Work out the finished part from the listing and answer in its coordinate system (mm). A direction names the side the tool comes from. Coordinates: 2 decimals unless noted, no trailing zeros. Order: outer loops, then holes, each group sorted by start corner. A loop starts at its lowest first (then second) coordinate and runs counter-clockwise, first axis right, second up.
1. The part is cut by section A-A, the plane z = -191. Give the vertices of the cut face in (x, y), then the cut area to 3 significant figures.
2. Flat-ended cylindrical pins translate along their axes: pin 1 Ø12 at (x, z) = (14, 3.5) entering from -Y; pin 2 Ø3 at (y, z) = (-79.5, -268.5) entering from -X; pin 3 Ø1.5 at (y, z) = (80, -9) entering from -X. Find the tip coordinate at first contact, or state that the pin passes through.
3. A tool of negligible diameter and unlimited length cuts with its end or side. For faces 1 (the flat face through (-345, -50, -250.774)), 2 (the flat face through (-38.1, -51, -160)), 3 (the flat face through (10, 85, 0)), 4 (the flat face through (-660.4, -50, -127)), 5 (the flat face through (-139.7, -18, -33)), from which of +Z, -Z, +X, -X, +Y, -Y can it reach the whole face along a straight path? Write none if from no direction.
4. The part is cut by section D-D, the plane x = -434.5. Give the vertices of the cut face in (y, z).
5. The part is cut by section B-B, the plane y = -45. Give the vertices of the cut face in (x, z).
6. Find the intervals of material crossed by probe 1 along X at (y, z) = (11, -62.5); probe 2 along Z at (x, y) = (-698.5, -65); probe 3 along X at (y, z) = (-39.5, -110), in increasing order.
7. Determine the mould class of faces 6 (the flat face through (10, 0, 84)), 7 (the flat face through (-165.1, -24, -24)), 8 (the flat face through (165.1, -1, -1)), 9 (the flat face through (-408, -76.2, -253)) for opening direction Y: +Y half, -Y half, draft (parallel to the pull), parting line (faces both ways), or undercut.
8. The part is cut by section C-C, the plane y = 55.5. Give the vertices of the cut face in (x, z), then the cut area to 3 significant figures.
```python
from build123d import *

# Parameters (mm, degrees)
F3_R      = 12.7
F4_DEPTH  = 50.8
F4_FACE_W = 76.2
F4_FACE_H = 50.8
F6_W      = 218.9167588949
F6_H      = 225.1323610544
F7_DEPTH  = 723.20793


with BuildPart() as f1:
    # F0 (on Front) → F1 (revolve)
    with BuildSketch(Plane.XZ):
        Polygon((165.1, 76.2), (165.1, 0), (190.5, 0), (190.5, 101.6), (-165.1, 101.6), (-165.1, 25.4), (-139.7, 25.4), (-139.7, 76.2), align=None)
    revolve(axis=Axis((0, 0, 0), (1, 0, 0)))

    # F3 (on offset) → F4 (join)
    with BuildSketch(Plane.XZ.offset(25.4)):
        with BuildLine():
            Line((38.1, -98.3737769937), (-38.1, -98.3737769937))
            Line((-38.1, -98.3737769937), (-38.1, -250.7737769937))
            Line((-38.1, -250.7737769937), (-660.4, -250.7737769937))
            Line((-660.4, -250.7737769937), (-660.4, 0))
            ThreePointArc((-660.4, 0), (-671.5592316368, 26.9407683632), (-698.5, 38.1))
            ThreePointArc((-698.5, 38.1), (-725.4407683632, 26.9407683632), (-736.6, 0))
            Line((-736.6, 0), (-736.6, -326.9737769937))
            Line((-736.6, -326.9737769937), (-660.4, -326.9737769937))
            Line((-660.4, -326.9737769937), (38.1, -326.9737769937))
            Line((38.1, -326.9737769937), (38.1, -250.7737769937))
            Line((38.1, -250.7737769937), (38.1, -98.3737769937))
        make_face()
        with Locations((-698.5, 0)):
            Circle(F3_R, mode=Mode.SUBTRACT)
    extrude(amount=F4_DEPTH)

    # F4_face (on face) → F5 (join, up to the next surface of F1)
    with BuildSketch(Plane(origin=(0, -50.8, -98.3737769937), x_dir=(1, 0, 0), z_dir=(0, 0, 1))):
        Rectangle(F4_FACE_W, F4_FACE_H)
    extrude(until=Until.NEXT)

    # F6 (on face) → F7 (cut)
    with BuildSketch(Plane(origin=(-165.1, 0, 0), x_dir=(0, -1, 0), z_dir=(-1, 0, 0))):
        with Locations((-109.4583794475, 112.5661805272)):
            Rectangle(F6_W, F6_H)
    extrude(amount=-F7_DEPTH, mode=Mode.SUBTRACT)


solid = f1.part
```
Geometry says:
1. outline: (-736.6, -76.2) - (-660.4, -76.2) - (-660.4, -25.4) - (-736.6, -25.4) - close; (-38.1, -76.2) - (38.1, -76.2) - (38.1, -25.4) - (-38.1, -25.4) - close
1. area: 7,740 mm2
2. pin 1: stops at y = -101.6
2. pin 2: passes through
2. pin 3: stops at x = -165.1
3. face 1: +Y, -Y
3. face 2: -Y
3. face 3: +Z, +X, -X, +Y
3. face 4: +Z, +Y, -Y
3. face 5: none
4. outline: (-76.2, -326.97) - (-25.4, -326.97) - (-25.4, -250.77) - (-76.2, -250.77) - close
5. outline: (-736.6, -326.97) - (38.1, -326.97) - (38.1, -91.09) - (190.5, -91.09) - (190.5, 91.09) - (-165.1, 91.09) - (-165.1, -91.09) - (-38.1, -91.09) - (-38.1, -250.77) - (-660.4, -250.77) - (-660.4, 0) arc R38.1 ccw to (-736.6, 0) - close; hole circle Ø25.4 at (-698.5, 0); hole (-139.7, -61.49) - (165.1, -61.49) - (165.1, 61.49) - (-139.7, 61.49) - close
6. probe 1: x = -165.1 to -139.7, 165.1 to 190.5
6. probe 2: z = -326.97 to -12.7, 12.7 to 38.1
6. probe 3: x = -736.6 to -660.4, -38.1 to 38.1
7. face 6: +Y half
7. face 7: draft
7. face 8: undercut
7. face 9: -Y half
8. outline: (-165.1, -85.1) - (190.5, -85.1) - (190.5, 0) - (165.1, 0) - (165.1, -52.21) - (-139.7, -52.21) - (-139.7, 0) - (-165.1, 0) - close
8. area: 14,300 mm2
